from build123d import *

# Parameters (mm, degrees)
SKETCH_2_W          = 180
SKETCH_2_H          = 120
EXTRUDE_1_DEPTH     = 3
FILLET_1_R          = 3.5
SKETCH_3_R          = 1.75
CUT_EXTRUDE_1_DEPTH = 4
SKETCH_4_R          = 1.75
CUT_EXTRUDE_2_DEPTH = 4


with BuildPart() as part:
    # 草图2 → 凸台-拉伸1 (new body)
    with BuildSketch(Plane(origin=(0, 0, 0), x_dir=(1, 0, 0), z_dir=(0, 1, 0))):
        with Locations((90, -60)):
            Rectangle(SKETCH_2_W, SKETCH_2_H)
    extrude(amount=EXTRUDE_1_DEPTH)

    # 圆角1
    fillet_1_edges = [part.edges().sort_by_distance(p)[0] for p in [
        (0, 1.5, 0),
        (180, 1.5, 0),
        (180, 1.5, 120),
        (0, 1.5, 120),
    ]]
    fillet(fillet_1_edges, radius=FILLET_1_R)

    # 草图3 → 切除-拉伸1 (cut, through all)
    with BuildSketch(Plane(origin=(0, 3, 0), x_dir=(1, 0, 0), z_dir=(0, 1, 0))):
        with Locations((175, -110.5)):
            Circle(SKETCH_3_R)
        with Locations((145, -110.5)):
            Circle(SKETCH_3_R)
        with Locations((175, -86.5)):
            Circle(SKETCH_3_R)
        with Locations((145, -86.5)):
            Circle(SKETCH_3_R)
    extrude(amount=-CUT_EXTRUDE_1_DEPTH, mode=Mode.SUBTRACT)

    # 草图4 → 切除-拉伸2 (cut, through all)
    with BuildSketch(Plane(origin=(0, 3, 0), x_dir=(1, 0, 0), z_dir=(0, 1, 0))):
        with Locations((110, -110)):
            Circle(SKETCH_4_R)
        with Locations((110, -10)):
            Circle(SKETCH_4_R)
        with Locations((10, -10)):
            Circle(SKETCH_4_R)
        with Locations((10, -110)):
            Circle(SKETCH_4_R)
    extrude(amount=-CUT_EXTRUDE_2_DEPTH, mode=Mode.SUBTRACT)


solid = part.part
Work out the finished part from the listing and answer in its coordinate system (mm). Give positions to 0.01 mm unless a question says otherwise; leave off trailing zeros. Write each loop counter-clockwise with the first axis right and the second up, starting at its lowest first coordinate (ties: lowest second). Pieces come first, ordered by that corner, then holes.
Q1. The part is cut by section B-B on z = 86.5. Give the vertices of the cut face in (x, y), and give its area (3 significant figures).
Answer:
outline: (0, 0) - (143.25, 0) - (143.25, 3) - (0, 3) - close; (146.75, 0) - (173.25, 0) - (173.25, 3) - (146.75, 3) - close; (176.75, 0) - (180, 0) - (180, 3) - (176.75, 3) - close
area: 519 mm2
Q2. For a pull along Z with two mould halves and no side action, classify faces 1 (the face through (176.669, 1.521, 85.974)), 2 (the face through (9.772, 1.521, 108.265)), 3 (the face through (178.95, 1.52, 119)), 4 (the face through (89, 3, 59)) as released by +Z, released by -Z, zero draft, split by the parting line, or undercut.
Answer:
face 1: undercut
face 2: undercut
face 3: released by +Z
face 4: zero draft
Q3. Straight lines are drawn through the part: L1, parallel to Z at x = 175, y = 1.05; L2, parallel to X at y = 2.3, z = 86.5; L3, parallel to Z at x = 110, y = 1.7. For each, find the intervals that lie inside material, in ascending order.
Answer:
L1: z = 0 to 84.75, 88.25 to 108.75, 112.25 to 120
L2: x = 0 to 143.25, 146.75 to 173.25, 176.75 to 180
L3: z = 0 to 8.25, 11.75 to 108.25, 111.75 to 120
Q4. The part is cut by section A-A on x = 10. Give the vertices of the cut face in (y, z).
Answer:
outline: (0, 0) - (3, 0) - (3, 8.25) - (0, 8.25) - close; (0, 11.75) - (3, 11.75) - (3, 108.25) - (0, 108.25) - close; (0, 111.75) - (3, 111.75) - (3, 120) - (0, 120) - close
